For this review, use the dimensioned drawing (mm, ordinates from the lowest corner) and the shaded views. A direction names the side the tool comes from. Coordinates: 2 decimals unless noted, no trailing zeros. Loops run counter-clockwise (first coordinate to the right, second up) from the corner with the lowest first, then second, coordinate; pieces in that order, holes last. Notation, with made-up numbers: (19, 66) - (35, 66) arc R37 cw to (35, 104) - close; hole circle Ø9 at (76.5, 10.5). An arc over 180 degrees is marked (long way). Answer in a Markdown table with one row per item. Add a question column.
(1) We need section D-D on y = 61.5. Write out the cut boundary in (x, z) (1 decimal).
(2) For P1, Ø10, axis at y = 46.5, z = 21, coming from the -X side; P2, Ø4, axis at y = 65.5, z = 7.5, coming from the -X side (1 decimal); P3, Ø12, axis at x = 52.5, y = 17.5, coming from the -Z side, all flat-tipped, find the tip position at first contact; note any pin that passes through.
(3) Machinability: for the marked faces 1, 2 and 3, which of the approach directions +Z, -Z, +X, -X, +Y, -Y give a long, thin tool a straight path to every point of the face, cutting with its end or side? Answer none if there is none.
(4) We need section B-B on z = 15.5. Write out the cut boundary in (x, y) (1 decimal).
(5) Mouldability with a two-part tool opening along Y and no side actions: class the marked faces 4, 5 and 6 as +Y half, -Y half, draft (parallel to the pull), parting line (faces both ways), or undercut.
(6) For line 1 along Y through (x, z) = (112, 7.5) (1 decimal); line 2 along X through (y, z) = (38, 12.75) (1 decimal); line 3 along Y through (x, z) = (97.5, 2.75) (1 decimal), list the stretches that pass through material, from the lowest coordinate up.
(7) We need section C-C on x = 32.5. Write out the cut boundary in (y, z) (1 decimal).
(8) We need section A-A on z = 7.5. Write out the cut boundary in (x, y) (1 decimal).
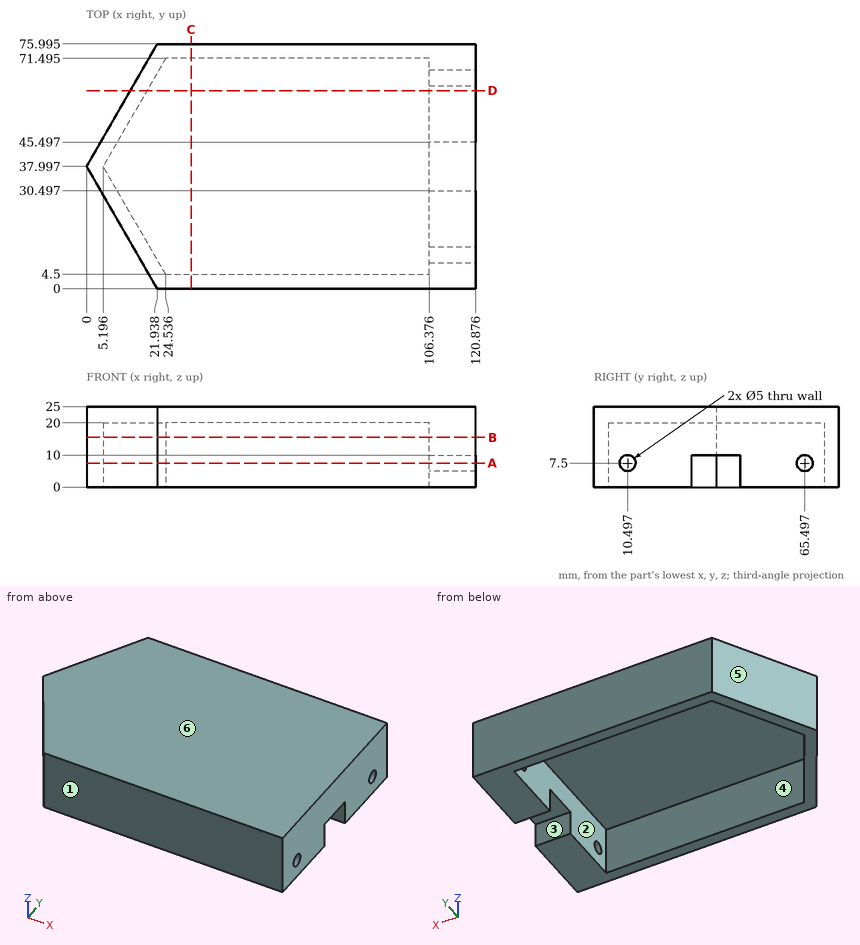
Outcome:
| question | item | result |
|---|---|---|
| 1 | outline | (13.6, 0) - (18.8, 0) - (18.8, 20) - (106.4, 20) - (106.4, 0) - (120.9, 0) - (120.9, 25) - (13.6, 25) - close |
| 2 | P1 | x = 2.02 |
| 2 | P2 | x = 14.7 |
| 2 | P3 | z = 20 |
| 3 | face 1 | +Z, -Z, +X, -X, -Y |
| 3 | face 2 | -Z |
| 3 | face 3 | -Z, +X |
| 4 | outline | (0, 38) - (21.9, 0) - (120.9, 0) - (120.9, 76) - (21.9, 76) - close; hole (5.2, 38) - (24.5, 4.5) - (106.4, 4.5) - (106.4, 71.5) - (24.5, 71.5) - close |
| 5 | face 4 | undercut |
| 5 | face 5 | +Y half |
| 5 | face 6 | draft |
| 6 | line 1 | 0 to 8, 13 to 30.5, 45.5 to 63, 68 to 76 |
| 6 | line 2 | 0 to 5.2, 106.4 to 120.9 |
| 6 | line 3 | 0 to 4.5, 71.5 to 76 |
| 7 | outline | (0, 0) - (4.5, 0) - (4.5, 20) - (71.5, 20) - (71.5, 0) - (76, 0) - (76, 25) - (0, 25) - close |
| 8 | outline | (0, 38) - (21.9, 0) - (120.9, 0) - (120.9, 8) - (106.4, 8) - (106.4, 4.5) - (24.5, 4.5) - (5.2, 38) - (24.5, 71.5) - (106.4, 71.5) - (106.4, 68) - (120.9, 68) - (120.9, 76) - (21.9, 76) - close; (106.4, 13) - (120.9, 13) - (120.9, 30.5) - (106.4, 30.5) - close; (106.4, 45.5) - (120.9, 45.5) - (120.9, 63) - (106.4, 63) - close |
